For this review, take the finished solid that the model builds, in its own axes (mm). Face numbers are marked on the shaded views. A direction names the side the tool comes from. Coordinates: 2 decimals unless noted, no trailing zeros. Loops run counter-clockwise (first coordinate to the right, second up) from the corner with the lowest first, then second, coordinate; pieces in that order, holes last. Notation, with made-up numbers: (42, -10) - (86, -10) arc R24 cw to (86, 6) - close; hole circle Ø7 at (20.25, 88). An arc over 180 degrees is marked (long way). One line per item, written item: value. Start each with the question number.
1. Take a section at B-B, the plane z = -16. State the section outline as (x, y) points.
2. Insertion check: pin 1 (9.5 mm diameter, centred on x = -8.5, z = 15, fed in from +Y); pin 2 (2 mm diameter, centred on x = 8.5, z = 0.5, fed in from -Y); pin 3 (8.5 mm diameter, centred on x = 7.5, y = 15.5, fed in from -Z). Each pin has a flat end and moves straight along its axis. Give the tip position at first contact, or say it passes through.
3. The part is to be moulded in two halves that separate along Y. For the marked faces 1, 2 and 3, say which applies: released by +Y, released by -Y, zero draft, split by the parting line, or undercut.
4. For the marked faces 4, 5, 6, 7 and 8, list the 3-axis set-ups (+Z, -Z, +X, -X, +Y, -Y) from which the entire face can be reached by the end or side of a thin tool; tool diameter is ignored.
5. To check wall thickness, follow line 1 (Y direction, x = -30, z = 0); line 2 (Z direction, x = -15.5, y = 29.5); line 3 (X direction, y = 3, z = -19.5). State the ranges of each line that lie inside material, in increasing order. Write a range as from..to.
6. Take a section at A-A, the plane x = -1.5. State the section outline as (y, z) points, and give its area (3 significant figures).
7. Take a section at D-D, the plane z = 3. State the section outline as (x, y) points, and give its area (3 significant figures).
8. Take a section at C-C, the plane y = 15. State the section outline as (x, z) points, and give its area (3 significant figures).
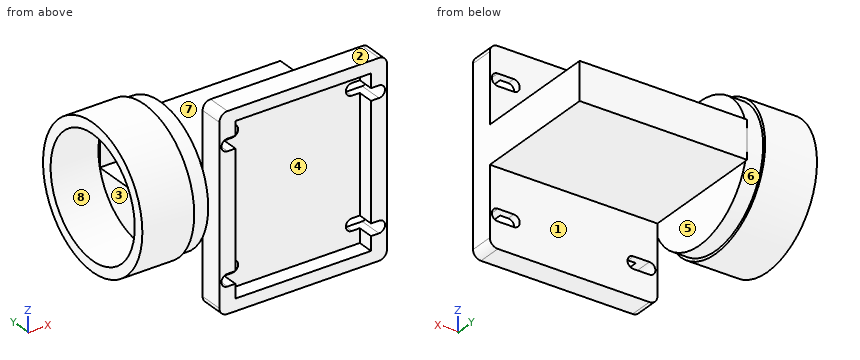
Autodesk Inventor part; units mm, degrees
ref_plane "YZ Plane" through (0, 0, 0) normal (1, 0, 0) x (0, 1, 0)
ref_plane "XZ Plane" through (0, 0, 0) normal (0, 1, 0) x (-1, 0, 0)
ref_plane "XY Plane" through (0, 0, 0) normal (0, 0, 1) x (1, 0, 0)
sketch "Sketch1" plane through (0, 0, 0) normal (0, 1, 0) x (-1, 0, 0)
  line L0 (29.9799, 0) -> (-29.9799, 0)
  line L1 (0, -34.1799) -> (0, 34.1799)
  line L2 (19, 24) -> (-19, 24)
  line L3 (-21, 22) -> (-21, -22)
  line L4 (-19, -24) -> (19, -24)
  line L5 (21, -22) -> (21, 22)
  arc A0 (21, 22) -> (19, 24) centre (19, 22) ccw
  arc A1 (19, -24) -> (21, -22) centre (19, -22) ccw
  arc A2 (-21, -22) -> (-19, -24) centre (-19, -22) ccw
  arc A3 (-19, 24) -> (-21, 22) centre (-19, 22) ccw
  point P0 (0, 0)
  point P1 (21, 24)
  point P2 (-21, -24)
  point P3 (-21, 24)
  point P4 (21, -24)
  dimension "d0" = 42
  dimension "d1" = 48
  dimension "d4" = 2
extrude "Extrusion1" add sketch "Sketch1" along normal blind 6
sketch "Sketch2" plane through (0, 0, 0) normal (0, -1, 0) x (1, 0, 0)
  line L0 (-29.4, 0) -> (29.4, 0)
  line L1 (0, -33.6) -> (0, 33.6)
  line L2 (17, 21) -> (-17, 21)
  line L3 (-17, 21) -> (-17, -21)
  line L4 (-17, -21) -> (17, -21)
  line L5 (17, -21) -> (17, 21)
  point P0 (0, 0)
  dimension "d5" = 34
  dimension "d6" = 42
extrude "Extrusion2" cut sketch "Sketch2" against normal blind 4
sketch "Sketch3" plane through (0, 6, 0) normal (0, 1, 0) x (1, 0, 0)
  line L0 (-29.4, 0) -> (29.4, 0)
  line L1 (0, 33.6) -> (0, -33.6)
  line L2 (19, 16) -> (15, 16) construction
  line L3 (17, -21) -> (17, 21)
  line L4 (19, 17.5) -> (15, 17.5)
  line L5 (15, 14.5) -> (19, 14.5)
  arc A0 (19, 14.5) -> (19, 17.5) centre (19, 16) ccw
  arc A1 (15, 17.5) -> (15, 14.5) centre (15, 16) ccw
  line L6 (19, 16) -> (23, 16) construction
  line L7 (21, -22) -> (21, 22)
  line L8 (19, 24) -> (-19, 24)
  point P0 (0, 0)
  point P1 (17, 16)
  dimension "d9" = 4
  dimension "d10" = 180
  dimension "d11" = 3
  dimension "d12" = 4
  dimension "d13" = 8
extrude "Extrusion3" cut sketch "Sketch3" against normal through all
mirror "Mirror1" about plane through (0, 0, 0) normal (0, 0, 1) of "Extrusion3"
mirror "Mirror2" about plane through (0, 0, 0) normal (1, 0, 0) of "Extrusion3", "Mirror1"
sketch "Sketch4" plane through (0, 6, 0) normal (0, 1, 0) x (1, 0, 0)
  line L0 (21, 4.75) -> (-21, 4.75)
  line L1 (-21, 4.75) -> (-21, -4.75)
  line L2 (-21, -4.75) -> (21, -4.75)
  line L3 (21, -4.75) -> (21, 4.75)
  line L4 (21, -22) -> (21, 22)
  line L5 (-21, 22) -> (-21, -22)
  line L6 (-29.4, 0) -> (29.4, 0)
  point P0 (0, 0)
  dimension "d16" = 9.5
extrude "Extrusion4" add sketch "Sketch4" along normal blind 32
sketch "Sketch5" plane through (-21, 0, -22) normal (-1, 0, 0) x (0, 0, 1)
  circle A0 centre (22, 21) radius 17
  line L0 (17.25, 38) -> (26.75, 38)
  line L1 (22, -7.6) -> (22, 45.6)
  point P0 (22, 0)
  dimension "d19" = 34
extrude "Extrusion5" add sketch "Sketch5" along normal blind 4
sketch "Sketch6" plane through (-25, 21, 0) normal (-1, 0, 0) x (0, 0, 1)
  circle A0 centre (0, 0) radius 17
  circle A1 centre (0, 0) radius 17.7
  point P0 (0, -21)
  dimension "d22" = 35.4
extrude "Extrusion6" add sketch "Sketch6" along normal blind 13 contours A0 | A1
sketch "Sketch7" plane through (-38, 21, 0) normal (-1, 0, 0) x (0, 0, 1)
  circle A0 centre (0, 0) radius 17.7
  circle A1 centre (0, 0) radius 15
  point P0 (0, -21)
  dimension "d25" = 30
extrude "Extrusion7" cut sketch "Sketch7" against normal blind 12 contours A1
sketch "Sketch8" plane through (-26, 21, 0) normal (-1, 0, 0) x (0, 0, 1)
  line L0 (-3.75, 14.5237) -> (3.75, 14.5237)
  line L1 (3.75, 14.5237) -> (3.75, -13.9763)
  line L2 (3.75, -13.9763) -> (-3.75, -13.9763)
  line L3 (-3.75, -13.9763) -> (-3.75, 14.5237)
  circle A0 centre (0, 0) radius 15
  line L4 (0, -28.74) -> (0, 25.44)
  point P0 (0, -21)
  dimension "d28" = 7.5
  dimension "d29" = 28.5
extrude "Extrusion8" cut sketch "Sketch8" against normal blind 45 contours L0 L4 L2 L3 | L0 L1 L2 L4
properties part number "boquilla_capnografo_V1"
Solutions:
1. outline: (-38, 13.43) - (-25, 13.43) - (-25, 15.26) - (-21, 15.26) - (-21, 26.74) - (-25, 26.74) - (-25, 28.57) - (-38, 28.57) - close; (-21, 0) - (-20.5, 0) - (-20.5, 6) - (-21, 6) - close; (-13.5, 4) - (13.5, 4) - (13.5, 6) - (-13.5, 6) - close; (20.5, 0) - (21, 0) - (21, 6) - (20.5, 6) - close
2. pin 1: y = 6
2. pin 2: y = 4
2. pin 3: z = -4.75
3. face 1: released by +Y
3. face 2: zero draft
3. face 3: undercut
4. face 4: -Y
4. face 5: -Z, +X, +Y
4. face 6: none
4. face 7: +Z, +X, +Y
4. face 8: -X
5. line 1: 3.3..6, 36..38.7
5. line 2: -4.75..-3.75, 3.75..4.75
5. line 3: -21..-17, 17..21
6. outline: (0, -24) - (6, -24) - (6, -4.75) - (38, -4.75) - (38, 4.75) - (6, 4.75) - (6, 24) - (0, 24) - (0, 21) - (4, 21) - (4, -21) - (0, -21) - close; hole (7.02, -3.75) - (35.52, -3.75) - (35.52, 3.75) - (7.02, 3.75) - close
6. area: 210 mm2
7. outline: (-38, 3.56) - (-25, 3.56) - (-25, 4.27) - (-21, 4.27) - (-21, 0) - (-17, 0) - (-17, 4) - (17, 4) - (17, 0) - (21, 0) - (21, 38) - (-21, 38) - (-21, 37.73) - (-25, 37.73) - (-25, 38.44) - (-38, 38.44) - (-38, 35.7) - (-26, 35.7) - (-26, 35.52) - (19, 35.52) - (19, 7.02) - (-26, 7.02) - (-26, 6.3) - (-38, 6.3) - close
7. area: 412 mm2
8. outline: (-38, -16.65) - (-25, -16.65) - (-25, -15.91) - (-21, -15.91) - (-21, -4.75) - (21, -4.75) - (21, 4.75) - (-21, 4.75) - (-21, 15.91) - (-25, 15.91) - (-25, 16.65) - (-38, 16.65) - (-38, 13.75) - (-26, 13.75) - (-26, 3.75) - (19, 3.75) - (19, -3.75) - (-26, -3.75) - (-26, -13.75) - (-38, -13.75) - close
8. area: 292 mm2
